from build123d import *

# Parameters (mm, degrees)
SKETCH1_R           = 20
SKETCH1_R_2         = 8
BOSS_EXTRUDE1_DEPTH = 10
FILLET1_R           = 4.5
SKETCH2_R           = 9
CUT_EXTRUDE1_DEPTH  = 2
SKETCH5_R           = 11
CUT_EXTRUDE2_DEPTH  = 2


with BuildPart() as part:
    # Sketch1 → Boss-Extrude1 (new body)
    with BuildSketch(Plane.XY):
        Circle(SKETCH1_R)
        Circle(SKETCH1_R_2, mode=Mode.SUBTRACT)
    extrude(amount=BOSS_EXTRUDE1_DEPTH)

    # Fillet1
    fillet1_edges = [part.edges().sort_by_distance(p)[0] for p in [
        (-20, 0, 0),
        (-20, 0, 10),
    ]]
    fillet(fillet1_edges, radius=FILLET1_R)

    # Sketch2 → Cut-Extrude1 (cut)
    with BuildSketch(Plane(origin=(0, 0, 0), x_dir=(-1, 0, 0), z_dir=(0, 0, -1))):
        Circle(SKETCH2_R)
    extrude(amount=-CUT_EXTRUDE1_DEPTH, mode=Mode.SUBTRACT)

    # Sketch5 → Cut-Extrude2 (cut)
    with BuildSketch(Plane.XY.offset(10)):
        Circle(SKETCH5_R)
    extrude(amount=-CUT_EXTRUDE2_DEPTH, mode=Mode.SUBTRACT)


solid = part.part
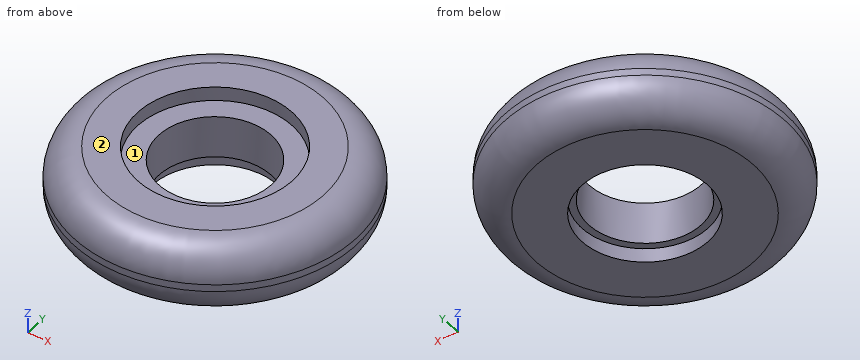
Work out the finished part from the listing and answer in its coordinate system (mm). Face numbers are marked on the shaded views. Round coordinates to 2 decimals unless told otherwise and drop trailing zeros. Order: outer loops, then holes, each group sorted by start corner. A loop starts at its lowest first (then second) coordinate and runs counter-clockwise, first axis right, second up. Notation, with made-up numbers: M 9,41 L 30,41 A15 ccw 30,62 Z; hole C 30.5,39 d5. An arc over 180 degrees is marked long. One line per item, written item: value.
Q1. Determine the mould class of the marked faces 1 and 2 for opening direction Y: released by +Y, released by -Y, zero draft, split by the parting line, or undercut.
Derived:
face 1: undercut
face 2: zero draft
Q2. Find section A-A on y = 0. Write down the section's boundary in (x, z), then the cut area to 3 significant figures.
Derived:
outline: M -20,4.5 A4.5 ccw -15.5,0 L -9,0 L -9,2 L -8,2 L -8,8 L -11,8 L -11,10 L -15.5,10 A4.5 ccw -20,5.5 Z; M 8,2 L 9,2 L 9,0 L 15.5,0 A4.5 ccw 20,4.5 L 20,5.5 A4.5 ccw 15.5,10 L 11,10 L 11,8 L 8,8 Z
area: 207 mm²
Q3. Find section D-D on z = 8.75. Write down the section's boundary in (x, y), then the cut area to 3 significant figures.
Derived:
outline: C 0,0 d37.22; hole C 0,0 d22
area: 708 mm²
Q4. Flat-ended cylindrical pins translate along their axes: pin 1 (20.5 mm diameter, centred on x = 0, y = 0, fed in from +Z); pin 2 (1 mm diameter, centred on y = 4.5, z = 8, fed in from -X); pin 3 (3 mm diameter, centred on y = -12, z = 8.5, fed in from +X). Find the tip coordinate at first contact, or state that the pin passes through.
Derived:
pin 1: z = 8
pin 2: x = -19.03
pin 3: x = 16.22
Q5. Straight lines are drawn through the part: line 1 (Y direction, x = 1.5, z = 6.25); line 2 (Y direction, x = 0, z = 8.6); line 3 (X direction, y = 7, z = 2.25). For each, find the intervals that lie inside material, in ascending order.
Derived:
line 1: -19.88 to -7.86, 7.86 to 19.88
line 2: -18.76 to -11, 11 to 18.76
line 3: -18.09 to -3.87, 3.87 to 18.09
Q6. Find section C-C on z = 1.25. Write down the section's boundary in (x, y), then the cut area to 3 significant figures.
Derived:
outline: C 0,0 d37.22; hole C 0,0 d18
area: 834 mm²
